```python
from build123d import *

# Parameters (mm, degrees)
BOSS_EXTRUDE1_DEPTH = 3


with BuildPart() as part:
    # Sketch3 → Boss-Extrude1 (new body)
    with BuildSketch(Plane(origin=(0, 0, 0), x_dir=(1, 0, 0), z_dir=(0, 1, 0))):
        with BuildLine():
            Line((-13.694996915, 20.301363277), (-15.860247962, 17.20906431))
            ThreePointArc((-15.860247962, 17.20906431), (-13.666207185, 14.707240293), (-12.875283017, 11.475))
            ThreePointArc((-12.875283017, 11.475), (-10.090653959, 8.727908609), (-6.180286102, 8.826363277))
            ThreePointArc((-6.180286102, 8.826363277), (0, 10.775), (6.180286102, 8.826363277))
            ThreePointArc((6.180286102, 8.826363277), (10.090653959, 8.727908609), (12.875283017, 11.475))
            ThreePointArc((12.875283017, 11.475), (13.666207185, 14.707240293), (15.860247962, 17.20906431))
            Line((15.860247962, 17.20906431), (13.694996915, 20.301363277))
            ThreePointArc((13.694996915, 20.301363277), (19.875283017, 22.25), (26.055569119, 20.301363277))
            Line((26.055569119, 20.301363277), (26.055569119, 31.138046441))
            ThreePointArc((26.055569119, 31.138046441), (21.514872246, 27.619726518), (15.870079226, 28.68406431))
            ThreePointArc((15.870079226, 28.68406431), (10.616247764, 27.083629141), (7, 22.95))
            ThreePointArc((7, 22.95), (0, 15.95), (-7, 22.95))
            ThreePointArc((-7, 22.95), (-10.616247764, 27.083629141), (-15.870079226, 28.68406431))
            ThreePointArc((-15.870079226, 28.68406431), (-21.514872246, 27.619726518), (-26.055569119, 31.138046441))
            Line((-26.055569119, 31.138046441), (-26.055569119, 20.301363277))
            ThreePointArc((-26.055569119, 20.301363277), (-19.875283017, 22.25), (-13.694996915, 20.301363277))
        make_face()
    extrude(amount=BOSS_EXTRUDE1_DEPTH)


solid = part.part
```
Here's how the part is built. I have some questions about the finished solid (model axes, mm). A direction names the side the tool comes from. Round coordinates to 2 decimals unless told otherwise and drop trailing zeros. Order: outer loops, then holes, each group sorted by start corner. A loop starts at its lowest first (then second) coordinate and runs counter-clockwise, first axis right, second up. Notation, with made-up numbers: M -4.75,48 L 43.25,48 A6 ccw 43.25,56 Z; hole C 29.25,57 d9. An arc over 180 degrees is marked long. Answer in a Markdown table with one row per item.
Item 1: Thinking about a two-plate mould opening in Z: for faces 4 (the face through (14.793, 1.479, -18.734)), 5 (the face through (-10.55, 1.48, -27.04)), 6 (the face through (-26.056, 1, -26)), which applies, +Z half, -Z half, draft (parallel to the pull), parting line (faces both ways), or undercut?
A:
| item | result |
|---|---|
| face 4 | undercut |
| face 5 | -Z half |
| face 6 | draft |
Item 2: Imagine slicing it at C-C, the plane x = 0. Write out the boundary of the cut face in (y, z) (3 decimals), and give its area (3 significant figures).
A:
| item | result |
|---|---|
| outline | M 0,-15.95 L 3,-15.95 L 3,-10.775 L 0,-10.775 Z |
| area | 15.5 mm2 |
Item 3: If I drill on L1, parallel to X at y = 0.55, z = -24.25; L2, parallel to Z at x = -23, y = 1.65; L3, parallel to X at y = 2.3, z = -19, over which ranges is the centre line in solid material (lowest first)? Write a range as from..to.
A:
| item | result |
|---|---|
| L1 | x = -26.06..-7.74, 7.74..26.06 |
| L2 | z = -28.16..-21.79 |
| L3 | x = -14.61..-5.78, 5.78..14.61 |
Item 4: Imagine slicing it at D-D, the plane z = -19.25. Write out the boundary of the cut face in (x, y).
A:
| item | result |
|---|---|
| outline | M -14.43,0 L -5.94,0 L -5.94,3 L -14.43,3 Z; M 5.94,0 L 14.43,0 L 14.43,3 L 5.94,3 Z |
Item 5: For faces 1 (the face through (10.682, 1.479, -27.126)), 2 (the face through (19.78, 1.48, -22.25)), 3 (the face through (0, 0, -15)), which set-ups out of +Z, -Z, +X, -X, +Y, -Y let a thin tool reach every point of the face, with its end or its side?
A:
| item | result |
|---|---|
| face 1 | -Z, +Y, -Y |
| face 2 | +Y, -Y |
| face 3 | +Z, -Z, +X, -X, -Y |
Item 6: Imagine slicing it at A-A, the plane z = -26.75. Write out the boundary of the cut face in (x, y), and give its area (3 significant figures).
A:
| item | result |
|---|---|
| outline | M -26.06,0 L -10.13,0 L -10.13,3 L -26.06,3 Z; M 10.13,0 L 26.06,0 L 26.06,3 L 10.13,3 Z |
| area | 95.5 mm2 |
Item 7: I'm going to push a flat-ended pin straight in: pin 1 (4 mm diameter, centred on x = 6.5, z = -26.5, fed in from -Y). Where does the tip first touch, or does it pass through?
A:
| item | result |
|---|---|
| pin 1 | passes through |
Item 8: Imagine slicing it at B-B, the plane y = 1.2. Write out the boundary of the cut face in (x, z) (3 decimals), and give its area (3 significant figures).
A:
| item | result |
|---|---|
| outline | M -26.056,-31.138 A7 cw -15.87,-28.684 A10 ccw -7,-22.95 A7 cw 7,-22.95 A10 ccw 15.87,-28.684 A7 cw 26.056,-31.138 L 26.056,-20.301 A10.775 cw 13.695,-20.301 L 15.86,-17.209 A7 cw 12.875,-11.475 A5 ccw 6.18,-8.826 A10.775 cw -6.18,-8.826 A5 ccw -12.875,-11.475 A7 cw -15.86,-17.209 L -13.695,-20.301 A10.775 cw -26.056,-20.301 Z |
| area | 507 mm2 |
